Verification items for the finished model (mm, model axes). A direction names the side the tool comes from. Coordinates: 2 decimals unless noted, no trailing zeros. Write each loop counter-clockwise with the first axis right and the second up, starting at its lowest first coordinate (ties: lowest second). Pieces come first, ordered by that corner, then holes. Notation, with made-up numbers: (63.5, -27.5) -> (88.5, -27.5) arc R30 ccw to (88.5, 1.5) -> close; hole circle Ø4 at (59, 10). An arc over 180 degrees is marked (long way). Write each question's results on one line, items separated by ' | '. Start each with the question number.
Autodesk Fusion 360 part; units mm, degrees
sketch "Esquisse1" plane through (0, 0, 0) normal (0, 0, 1) x (1, 0, 0)
  line L0 (0, 0) -> (35, 0)
  line L1 (35, 0) -> (35, 6)
  line L2 (35, 6) -> (0, 6)
  line L3 (0, 6) -> (0, 0)
  line L4 (7.5, 6) -> (27.5, 6)
  line L5 (27.5, 6) -> (27.5, 44)
  line L6 (27.5, 44) -> (7.5, 44)
  line L7 (7.5, 44) -> (7.5, 6)
  circle A0 centre (17.5, 34) radius 5
  line L8 (7.5, 44) -> (27.5, 44) construction
  line L9 (27.5, 44) -> (27.5, 24) construction
  line L10 (27.5, 24) -> (7.5, 24) construction
  line L11 (7.5, 24) -> (7.5, 44) construction
  line L12 (7.5, 44) -> (27.5, 24) construction
  line L13 (27.5, 44) -> (7.5, 24) construction
  dimension "d1" = 35
  dimension "d2" = 6
  dimension "d3" = 20
  dimension "d5" = 10
  dimension "d6" = 20
  dimension "d7" = 20
  dimension "d10" = 34
extrude "Extrusion1" add sketch "Esquisse1" along normal blind 8
sketch "Esquisse2" plane through (0, 6, 0) normal (0, 1, 0) x (-1, 0, 0)
  line L0 (-7.5, 0) -> (0, 0)
  line L1 (0, 0) -> (0, 8)
  line L2 (0, 8) -> (-7.5, 8)
  line L3 (-7.5, 8) -> (-7.5, 0)
  circle A0 centre (-3.75, 4) radius 2.1
  line L4 (0, 0) -> (-7.5, 8) construction
  line L5 (-7.5, 0) -> (0, 8) construction
  dimension "d11" = 4.2
sketch "Esquisse3" plane through (0, 6, 0) normal (0, 1, 0) x (-1, 0, 0)
  line L0 (-35, 0) -> (-27.5, 0)
  line L1 (-27.5, 0) -> (-27.5, 8)
  line L2 (-27.5, 8) -> (-35, 8)
  line L3 (-35, 8) -> (-35, 0)
  line L4 (-27.5, 0) -> (-35, 8) construction
  line L5 (-35, 0) -> (-27.5, 8) construction
  circle A0 centre (-31.25, 4) radius 2.1
  dimension "d12" = 4.2
extrude "Extrusion2" cut sketch "Esquisse2" sketch "Esquisse3" against normal blind 10 contours A0 of sketch 2 contours A0
fillet "Congé1" radius 0.5 2 edges at (5.7079, 0, 3.2406) (33.2079, 0, 3.2406)
fillet "Congé2" radius 5 2 edges at (7.5, 44, 4) (27.5, 44, 4)
1. Sectioned sample at A-A on x = 17.5. Record the cut outline in (y, z), plus the area to 3 significant figures.
2. Material ranges on probe 1 along Y at (x, z) = (17.5, 4.75); probe 2 along Y at (x, z) = (28, 3); probe 3 along Z at (x, y) = (31, 4), recorded low to high. Write a range as from..to.
3. Sectioned sample at B-B on y = 34. Record the cut outline in (x, z).
4. Sectioned sample at D-D on x = 3.75. Record the cut outline in (y, z), plus the area to 3 significant figures.
5. Tool access check on faces 4 (the flat face through (2, 6, 6)), 5 (the flat face through (27.5, 22, 4)), 6 (the cylindrical face through (33.35, 3.29, 4.09)). Record the directions out of +Z, -Z, +X, -X, +Y, -Y that give a thin tool (end or side, any length) a straight path to the whole face; none if there is none.
6. Depth check by flat-ended pin: pin 1 Ø1.5 at (y, z) = (24.5, 2) entering from +X; pin 2 Ø2 at (y, z) = (26.5, 1) entering from -X; pin 3 Ø2 at (x, z) = (2.5, 3.5) entering from +Y. Enter the tip coordinate at first touch or a pass-through.
7. Mould release check, pull along X, two halves, no side actions. Record for faces 1 (the flat face through (7.5, 23, 4)), 2 (the flat face through (33, 6, 6)), 3 (the cylindrical face through (16.42, 38.88, 3.94)): +X half, -X half, draft (parallel to the pull), parting line (faces both ways), or undercut.
8. Sectioned sample at C-C on z = 4.5. State how many separate pieces and enclosed holes the cut face has, plus the area to 3 significant figures.
Computed values:
1) outline: (0, 0) -> (29, 0) -> (29, 8) -> (0, 8) -> close; (39, 0) -> (44, 0) -> (44, 8) -> (39, 8) -> close | area: 272 mm^2
2) probe 1: y = 0..29, 39..44 | probe 2: y = 0..6 | probe 3: z = 0..1.91, 6.09..8
3) outline: (7.5, 0) -> (12.5, 0) -> (12.5, 8) -> (7.5, 8) -> close; (22.5, 0) -> (27.5, 0) -> (27.5, 8) -> (22.5, 8) -> close
4) outline: (0, 0) -> (6, 0) -> (6, 1.9) -> (0.5, 1.9) arc R0.5 ccw to (0, 1.4) -> close; (0, 6.6) arc R0.5 ccw to (0.5, 6.1) -> (6, 6.1) -> (6, 8) -> (0, 8) -> close | area: 22.7 mm^2
5) face 4: +Z, -Z, -X, +Y | face 5: +Z, -Z, +X, +Y | face 6: +Y, -Y
6) pin 1: stops at x = 27.5 | pin 2: stops at x = 7.5 | pin 3: stops at y = 6
7) face 1: -X half | face 2: draft | face 3: undercut
8) separate pieces: 3 | enclosed holes: 1 | area: 832 mm^2
